Work out the finished part from the listing and answer in its coordinate system (mm). A direction names the side the tool comes from. Coordinates: 2 decimals unless noted, no trailing zeros. Loops run counter-clockwise (first coordinate to the right, second up) from the corner with the lowest first, then second, coordinate; pieces in that order, holes last.
```python
from build123d import *

# Parameters (mm, degrees)
F1_DEPTH = 114.3
F2_START = 25.4
F2_DEPTH = 88.901
F3_R     = 25.4


with BuildPart() as f1:
    # F0 (on Top) → F1 (new body)
    with BuildSketch(Plane.XY):
        Polygon((508, 0), (-508, 0), (-508, -603.25), (-292.1, -603.25), (-252.9113285375, -381), (252.9113285375, -381), (292.1, -603.25), (508, -603.25), align=None)
        Polygon((-252.9113285375, -381), (-292.1, -603.25), (292.1, -603.25), (252.9113285375, -381), align=None)
    extrude(amount=F1_DEPTH)

    # F0 (on Top) → F2 (cut)
    with BuildSketch(Plane.XY.offset(F2_START)):
        Polygon((-252.9113285375, -381), (-292.1, -603.25), (292.1, -603.25), (252.9113285375, -381), align=None)
    extrude(amount=F2_DEPTH, mode=Mode.SUBTRACT)

    # F3
    f3_edges = [f1.edges().sort_by_distance(p)[0] for p in [
        (-508, -603.25, 57.15),
        (508, -603.25, 57.15),
        (-292.1, -603.25, 69.85),
        (-252.911329, -381, 69.85),
        (292.1, -603.25, 69.85),
        (508, 0, 57.15),
        (252.911329, -381, 69.85),
        (-508, 0, 57.15),
    ]]
    fillet(f3_edges, radius=F3_R)


solid = f1.part
```
1. Straight lines are drawn through the part: probe 1 along Z at (x, y) = (244, -486); probe 2 along Y at (x, z) = (49, 85); probe 3 along X at (y, z) = (-428, 90). For each, find the intervals that lie inside material, in ascending order.
2. Determine the mould class of faces 3 (the flat face through (-272.283, -490.863, 69.228)), 4 (the flat face through (-508, -298, 56)), 5 (the flat face through (-7, -603.25, 18)) for opening direction X: released by +X, released by -X, zero draft, split by the parting line, or undercut.
3. A cutting plane is placed at B-B, the plane y = -472. Give the vertices of the cut face in (x, z), then the cut area to 3 significant figures.
4. A cutting plane is placed at A-A, the plane z = 77.5. Give the vertices of the cut face in (x, y), then the cut area to 3 significant figures.
5. A cutting plane is placed at C-C, the plane x = -46. Give the vertices of the cut face in (y, z).
6. For faces 1 (the flat face through (-4, -491, 25.4)), 2 (the cylindrical face through (-500.76, -595.61, 57.95)), determine the directions among +Z, -Z, +X, -X, +Y, -Y from which every point of the face is accessible in a straight line to the end or side of a thin tool.
Answers below:
1. probe 1: z = 0 to 25.4
1. probe 2: y = -381 to 0
1. probe 3: x = -508 to -261.2, 261.2 to 508
2. face 3: undercut
2. face 4: released by -X
2. face 5: zero draft
3. outline: (-508, 0) - (508, 0) - (508, 114.3) - (268.96, 114.3) - (268.96, 25.4) - (-268.96, 25.4) - (-268.96, 114.3) - (-508, 114.3) - close
3. area: 68,300 mm2
4. outline: (-508, -577.85) arc R25.4 ccw to (-482.6, -603.25) - (-313.41, -603.25) arc R25.4 ccw to (-288.4, -582.26) - (-256.61, -401.99) arc R25.4 cw to (-231.6, -381) - (231.6, -381) arc R25.4 cw to (256.61, -401.99) - (288.4, -582.26) arc R25.4 ccw to (313.41, -603.25) - (482.6, -603.25) arc R25.4 ccw to (508, -577.85) - (508, -25.4) arc R25.4 ccw to (482.6, 0) - (-482.6, 0) arc R25.4 ccw to (-508, -25.4) - close
4. area: 491,000 mm2
5. outline: (-603.25, 0) - (0, 0) - (0, 114.3) - (-381, 114.3) - (-381, 25.4) - (-603.25, 25.4) - close
6. face 1: +Z, -Y
6. face 2: +Z, -Z, -X, -Y
